```python
from build123d import *

# Parameters (mm, degrees)
F0_R     = 25.077837
F0_R_2   = 13.665019
F1_DEPTH = 41.91
F2_SIZE  = 5.08
F3_R     = 5.08


with BuildPart() as f1:
    # F0 (on Top) → F1 (new body)
    with BuildSketch(Plane.XY):
        Circle(F0_R)
        Circle(F0_R_2, mode=Mode.SUBTRACT)
    extrude(amount=F1_DEPTH)

    # F2
    f2_edges = [f1.edges().sort_by_distance(p)[0] for p in [
        (-13.665019, 0, 41.91),
    ]]
    chamfer(f2_edges, length=F2_SIZE)

    # F3
    f3_edges = [f1.edges().sort_by_distance(p)[0] for p in [
        (-25.077837, 0, 41.91),
        (-25.077837, 0, 0),
    ]]
    fillet(f3_edges, radius=F3_R)


solid = f1.part
```
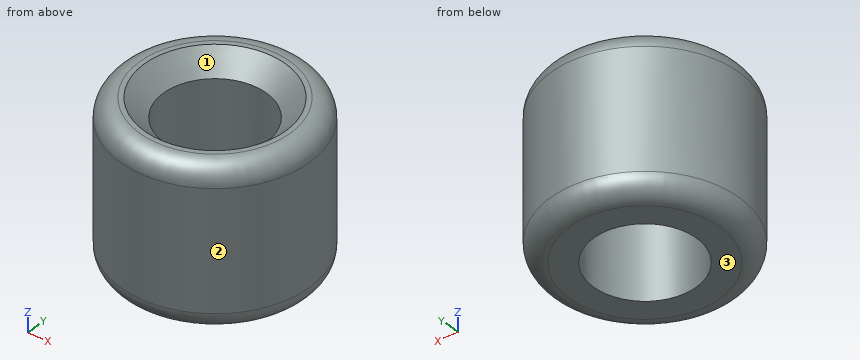
Build history of the part. All positions in model axes, mm. Face numbers are marked on the shaded views. Coordinates: 2 decimals unless noted, no trailing zeros. Write each loop counter-clockwise with the first axis right and the second up, starting at its lowest first coordinate (ties: lowest second). Pieces come first, ordered by that corner, then holes.
1. Pull direction X, two halves, no side cores. Call the marked faces 1, 2 and 3: released by +X, released by -X, zero draft, split by the parting line, or undercut.
Answer block:
face 1: undercut
face 2: split by the parting line
face 3: zero draft
2. Drop flat-ended pins along their axis: pin 1 (6 mm diameter, centred on x = -7.5, z = 6, fed in from +Y); pin 2 (6 mm diameter, centred on y = 18, z = 36, fed in from -X); pin 3 (1 mm diameter, centred on y = 7.5, z = 25.5, fed in from +X). Give the stop position or say it passes through.
Answer block:
pin 1: stops at y = 24.67
pin 2: stops at x = -20.1
pin 3: stops at x = 24.08
3. Band-saw the part on D-D, the plane z = 3. Give the cut face in (x, y), and give its area (3 significant figures).
Answer block:
outline: circle Ø49.26 at (0, 0); hole circle Ø27.33 at (0, 0)
area: 1,320 mm2
4. Drill centre lines: probe 1 along Y at (x, z) = (0, 22); probe 2 along X at (y, z) = (5.5, 29); probe 3 along Y at (x, z) = (-12.5, 13). Where is each one in solid material? Low to high.
Answer block:
probe 1: y = -25.08 to -13.67, 13.67 to 25.08
probe 2: x = -24.47 to -12.51, 12.51 to 24.47
probe 3: y = -21.74 to -5.52, 5.52 to 21.74
5. Band-saw the part on C-C, the plane z = 23. Give the cut face in (x, y), and give its area (3 significant figures).
Answer block:
outline: circle Ø50.16 at (0, 0); hole circle Ø27.33 at (0, 0)
area: 1,390 mm2
6. Band-saw the part on A-A, the plane x = 0. Give the cut face in (y, z).
Answer block:
outline: (-25.08, 5.08) arc R5.08 ccw to (-20, 0) - (-13.67, 0) - (-13.67, 36.83) - (-18.75, 41.91) - (-20, 41.91) arc R5.08 ccw to (-25.08, 36.83) - close; (13.67, 0) - (20, 0) arc R5.08 ccw to (25.08, 5.08) - (25.08, 36.83) arc R5.08 ccw to (20, 41.91) - (18.75, 41.91) - (13.67, 36.83) - close
